The listing builds one solid part. Answer for the finished solid, in the listing's coordinates (mm). A direction names the side the tool comes from. Round coordinates to 2 decimals unless told otherwise and drop trailing zeros. Loops run counter-clockwise (first coordinate to the right, second up) from the corner with the lowest first, then second, coordinate; pieces in that order, holes last. Notation, with made-up numbers: (59.5, -11) -> (87.5, -11) arc R7 ccw to (87.5, -5) -> close; hole circle Ø3 at (-9.75, 20). An arc over 180 degrees is marked (long way). Use a Markdown table: item, result. Add a question column.
Q1. Which of the six approach directions +Z, -Z, +X, -X, +Y, -Y give full straight-line access (tool end or side, diameter ignored) to faces 4 (the flat face through (-14.8, 3, 0)), 5 (the flat face through (15, 3, -8)), 6 (the flat face through (0, 3, -14.8))?
Q2. Given pin 1 Ø3 at (x, z) = (-1.5, 6) entering from +Y, flat-ended and moving along its own axis, determine where the tip first touches the part or whether it passes through.
Q3. For a pull along Z with two mould halves and no side action, classify faces 1 (the flat face through (0, 3, -15)), 2 (the flat face through (14.8, 3, 9)), 3 (the flat face through (0, 2, 0)) as released by +Z, released by -Z, zero draft, split by the parting line, or undercut.
Q4. Section A-A on y = 2.85 is taken. Give the vertices of the cut face in (x, z), then the cut area to 3 significant figures.
Q5. Section B-B on x = -6.5 is taken. Give the vertices of the cut face in (y, z), then the cut area to 3 significant figures.
Q6. Consider line 1 (Z direction, x = 7, y = 3.65); line 2 (Y direction, x = -7, z = -6.75). Determine where each line is inside the solid, lowest interval first.
Q7. Section C-C on z = -3 is taken. Give the vertices of the cut face in (x, y), then the cut area to 3 significant figures.
from build123d import *

# Parameters (mm, degrees)
BASES_W            = 29.4
BASES_H            = 29.4
BASE_DEPTH         = 0.2
EDGE_FLANGE1_DEPTH = 29.4
EDGE_FLANGE2_DEPTH = 29.4
EDGE_FLANGE3_DEPTH = 29.4
EDGE_FLANGE4_DEPTH = 29.4
VENT_DEPTH         = 42.363026969
VENT_DEPTH_BACK    = 42.363026969


# Sheet-metal steps are written as plain solids
with BuildPart() as part:
    # BaseS → Base (new body)
    with BuildSketch(Plane(origin=(0, 2, 0), x_dir=(1, 0, 0), z_dir=(0, 1, 0))):
        Rectangle(BASES_W, BASES_H)
    extrude(amount=-BASE_DEPTH)

    # Edge-Flange1 section (across the edge) → Edge-Flange1 (add)
    with BuildSketch(Plane(origin=(-14.7, 2, 14.8), x_dir=(0, 0, -1), z_dir=(1, 0, 0))):
        with BuildLine():
            Line((-0.2, 0.1), (-0.2, 1.8))
            Line((-0.2, 1.8), (0, 1.8))
            Line((0, 1.8), (0, 0.1))
            ThreePointArc((0, 0.1), (0.029289322, 0.029289322), (0.1, 0))
            Line((0.1, 0), (0.1, -0.2))
            ThreePointArc((0.1, -0.2), (-0.112132034, -0.112132034), (-0.2, 0.1))
        make_face()
    extrude(amount=EDGE_FLANGE1_DEPTH)

    # Edge-Flange2 section (across the edge) → Edge-Flange2 (add)
    with BuildSketch(Plane(origin=(14.7, 2, -14.8), x_dir=(0, 0, 1), z_dir=(-1, 0, 0))):
        with BuildLine():
            Line((-0.2, 0.1), (-0.2, 1.8))
            Line((-0.2, 1.8), (0, 1.8))
            Line((0, 1.8), (0, 0.1))
            ThreePointArc((0, 0.1), (0.029289322, 0.029289322), (0.1, 0))
            Line((0.1, 0), (0.1, -0.2))
            ThreePointArc((0.1, -0.2), (-0.112132034, -0.112132034), (-0.2, 0.1))
        make_face()
    extrude(amount=EDGE_FLANGE2_DEPTH)

    # Edge-Flange3 section (across the edge) → Edge-Flange3 (add)
    with BuildSketch(Plane(origin=(14.8, 2, 14.7), x_dir=(-1, 0, 0), z_dir=(0, 0, -1))):
        with BuildLine():
            Line((-0.2, 0.1), (-0.2, 1.8))
            Line((-0.2, 1.8), (0, 1.8))
            Line((0, 1.8), (0, 0.1))
            ThreePointArc((0, 0.1), (0.029289322, 0.029289322), (0.1, 0))
            Line((0.1, 0), (0.1, -0.2))
            ThreePointArc((0.1, -0.2), (-0.112132034, -0.112132034), (-0.2, 0.1))
        make_face()
    extrude(amount=EDGE_FLANGE3_DEPTH)

    # Edge-Flange4 section (across the edge) → Edge-Flange4 (add)
    with BuildSketch(Plane(origin=(-14.8, 2, -14.7), x_dir=(1, 0, 0), z_dir=(0, 0, 1))):
        with BuildLine():
            Line((-0.2, 0.1), (-0.2, 1.8))
            Line((-0.2, 1.8), (0, 1.8))
            Line((0, 1.8), (0, 0.1))
            ThreePointArc((0, 0.1), (0.029289322, 0.029289322), (0.1, 0))
            Line((0.1, 0), (0.1, -0.2))
            ThreePointArc((0.1, -0.2), (-0.112132034, -0.112132034), (-0.2, 0.1))
        make_face()
    extrude(amount=EDGE_FLANGE4_DEPTH)

    # VentS → Vent (cut, two sides: drawn at the far end of the back side and taken through both)
    with BuildSketch(Plane(origin=(-15.1, 1.8, -13.3), x_dir=(1, 0, 0), z_dir=(0, 1, 0)).offset(-VENT_DEPTH_BACK)):
        with BuildLine():
            Line((30.1, -11.05), (30.1, -15.55))
            Line((30.1, -15.55), (29.1, -15.55))
            ThreePointArc((29.1, -15.55), (28.746446609, -15.403553391), (28.6, -15.05))
            Line((28.6, -15.05), (28.6, -11.55))
            ThreePointArc((28.6, -11.55), (28.746446609, -11.196446609), (29.1, -11.05))
            Line((29.1, -11.05), (30.1, -11.05))
        make_face()
    extrude(amount=VENT_DEPTH + VENT_DEPTH_BACK, mode=Mode.SUBTRACT)


solid = part.part
Checked values:
| question | item | result |
|---|---|---|
| 1 | face 4 | +Z, -Z, +Y |
| 1 | face 5 | +Z, -Z, +X, +Y, -Y |
| 1 | face 6 | +X, -X, +Y |
| 2 | pin 1 | stops at y = 2 |
| 3 | face 1 | released by -Z |
| 3 | face 2 | zero draft |
| 3 | face 3 | undercut |
| 4 | outline | (-15, -14.7) -> (-14.8, -14.7) -> (-14.8, 14.7) -> (-15, 14.7) -> close; (-14.7, -15) -> (14.7, -15) -> (14.7, -14.8) -> (-14.7, -14.8) -> close; (-14.7, 14.8) -> (14.7, 14.8) -> (14.7, 15) -> (-14.7, 15) -> close; (14.8, -14.7) -> (15, -14.7) -> (15, -2.25) -> (14.8, -2.25) -> close; (14.8, 2.25) -> (15, 2.25) -> (15, 14.7) -> (14.8, 14.7) -> close |
| 4 | area | 22.6 mm2 |
| 5 | outline | (1.8, -14.7) arc R0.3 ccw to (2.1, -15) -> (3.8, -15) -> (3.8, -14.8) -> (2.1, -14.8) arc R0.1 cw to (2, -14.7) -> (2, 14.7) arc R0.1 cw to (2.1, 14.8) -> (3.8, 14.8) -> (3.8, 15) -> (2.1, 15) arc R0.3 ccw to (1.8, 14.7) -> close |
| 5 | area | 6.69 mm2 |
| 6 | line 1 | z = -15 to -14.8, 14.8 to 15 |
| 6 | line 2 | y = 1.8 to 2 |
| 7 | outline | (-15, 2.1) arc R0.3 ccw to (-14.7, 1.8) -> (14.7, 1.8) arc R0.3 ccw to (15, 2.1) -> (15, 3.8) -> (14.8, 3.8) -> (14.8, 2.1) arc R0.1 cw to (14.7, 2) -> (-14.7, 2) arc R0.1 cw to (-14.8, 2.1) -> (-14.8, 3.8) -> (-15, 3.8) -> close |
| 7 | area | 6.69 mm2 |
